Here's how the part is built. I have some questions about the finished solid (model axes, mm). A direction names the side the tool comes from. Give positions to 0.01 mm unless a question says otherwise; leave off trailing zeros. Loops run counter-clockwise (first coordinate to the right, second up) from the corner with the lowest first, then second, coordinate; pieces in that order, holes last.
Q1. Suppose I cut it at A-A (x = 0). List the corners of the cut face in (y, z) for me, and give its area (3 significant figures).
Q2. I need wall thicknesses on probe 1 along Y at (x, z) = (-57.5, 1.1) (3 decimals); probe 2 along X at (y, z) = (1.75, 2.5); probe 3 along Y at (x, z) = (15.5, 1.35). Which ranges of each line are inside material? Lowest first, please.
Q3. Suppose I cut it at D-D (y = 4.75). List the corners of the cut face in (x, z) for me, and give its area (3 significant figures).
Q4. Suppose I cut it at C-C (x = 10). List the corners of the cut face in (y, z) for me.
Q5. Suppose I cut it at B-B (z = 0.5). Count the separate pieces of the cut face and the enclosed holes in it, and give its area (3 significant figures).
Q6. I'm going to push flat-ended pins straight in: P1, Ø1.2, axis at x = -6.5, y = 0, coming from the +Z side; P2, Ø1.5, axis at y = -3, z = 2, coming from the +X side. Where does each tip first touch, or does it pass through?
Q7. For faces 5 (the face through (7, 0.75, 2)), 6 (the face through (-24, 0, 0)), which set-ups out of +Z, -Z, +X, -X, +Y, -Y let a thin tool reach every point of the face, with its end or its side?
Q8. Thinking about a two-plate mould opening in Y: for faces 1 (the face through (-24, 0, 3)), 2 (the face through (7, -0.75, 2)), 3 (the face through (-7, -0.75, 2)), 4 (the face through (21, 0, 1)), which applies, pulls with the +Y half, pulls with the -Y half, needs draft (parallel to the pull), parting line crosses it, or undercut?
```python
from build123d import *

# Parameters (mm, degrees)
SKETCH1_R               = 1.45
SKETCH1_R_2             = 2.95
BOSS_EXTRUDE1_DEPTH     = 3
TROU_TARAUD_M1_61_D     = 1.25
ESQUISSE3_W             = 22
ESQUISSE3_H             = 1.5
ENL_V_MAT_EXTRU_1_DEPTH = 1.6


with BuildPart() as part:
    # Sketch1 → Boss-Extrude1 (new body)
    with BuildSketch(Plane.XY):
        with BuildLine():
            Line((15.5, 5.5), (-62, 5.5))
            ThreePointArc((-62, 5.5), (-67.5, 0), (-62, -5.5))
            Line((-62, -5.5), (15.5, -5.5))
            ThreePointArc((15.5, -5.5), (21, 0), (15.5, 5.5))
        make_face()
        with Locations((-62, 0)):
            Circle(SKETCH1_R, mode=Mode.SUBTRACT)
        Circle(SKETCH1_R_2, mode=Mode.SUBTRACT)
        with Locations((15.5, 0)):
            Circle(SKETCH1_R_2, mode=Mode.SUBTRACT)
    extrude(amount=BOSS_EXTRUDE1_DEPTH)

    # Trou taraudé M1.61 (through all)
    with Locations(Plane.XY.offset(3)):
        with Locations((7.75, 2.5), (-7.75, 2.5), (-57.5, 2.5), (-50, 2.5)):
            trou_taraud_m1_61 = Hole(TROU_TARAUD_M1_61_D / 2)

    # Mirror1: Trou taraudé M1.61 across plane
    add(trou_taraud_m1_61.mirror(Plane.ZX), mode=Mode.SUBTRACT)

    # Esquisse3 → Enlèv. mat.-Extru.1 (cut)
    with BuildSketch(Plane.XY.offset(3)):
        Rectangle(ESQUISSE3_W, ESQUISSE3_H)
    extrude(amount=-ENL_V_MAT_EXTRU_1_DEPTH, mode=Mode.SUBTRACT)


solid = part.part
```
Solutions:
1. outline: (-5.5, 0) - (-2.95, 0) - (-2.95, 3) - (-5.5, 3) - close; (2.95, 0) - (5.5, 0) - (5.5, 3) - (2.95, 3) - close
1. area: 15.3 mm2
2. probe 1: y = -5.5 to -3.125, -1.875 to 1.875, 3.125 to 5.5
2. probe 2: x = -67.21 to -2.37, 2.37 to 13.13, 17.87 to 20.71
2. probe 3: y = -5.5 to -2.95, 2.95 to 5.5
3. outline: (-64.77, 0) - (18.27, 0) - (18.27, 3) - (-64.77, 3) - close
3. area: 249 mm2
4. outline: (-5.5, 0) - (5.5, 0) - (5.5, 3) - (0.75, 3) - (0.75, 1.4) - (-0.75, 1.4) - (-0.75, 3) - (-5.5, 3) - close
5. separate pieces: 1
5. enclosed holes: 11
5. area: 876 mm2
6. P1: stops at z = 1.4
6. P2: stops at x = 20.52
7. face 5: +Z
7. face 6: -Z, +X, -X, +Y, -Y
8. face 1: needs draft
8. face 2: undercut
8. face 3: undercut
8. face 4: parting line crosses it
